from build123d import *

# Parameters (mm, degrees)
SKETCH1_W           = 50.8
SKETCH1_H           = 95.25
BOSS_EXTRUDE1_DEPTH = 38.1
SKETCH2_W           = 74.255386752
SKETCH2_H           = 8.89
F_0_DEG_SLOT_DEPTH  = 19.05
SKETCH3_W           = 5.0292
SKETCH3_H           = 76.2
BOSS_EXTRUDE2_DEPTH = 6.35
SKETCH4_R           = 4.9022
CUT_EXTRUDE2_DEPTH  = 67.067470248
SKETCH5_R           = 5.842
CUT_EXTRUDE3_DEPTH  = 12.319
F_45DEG_SLOT_DEPTH  = 19.05
F_30_DEG_SLOT_DEPTH = 19.05
FILLET2_R           = 6.35
F_15_DEG_SLOT_DEPTH = 19.05
FILLET4_R           = 2.5146
FILLET3_R           = 1.27


with BuildPart() as part:
    # Sketch1 → Boss-Extrude1 (new body)
    with BuildSketch(Plane.XY):
        Rectangle(SKETCH1_W, SKETCH1_H)
    extrude(amount=BOSS_EXTRUDE1_DEPTH)

    # Sketch2 → 0 deg slot (cut)
    with BuildSketch(Plane.XY.offset(38.1)):
        Rectangle(SKETCH2_W, SKETCH2_H)
    extrude(amount=-F_0_DEG_SLOT_DEPTH, mode=Mode.SUBTRACT)

    # Sketch3 → Boss-Extrude2 (add)
    with BuildSketch(Plane(origin=(0, 0, 0), x_dir=(-1, 0, 0), z_dir=(0, 0, -1))):
        with Locations((-15, 0)):
            Rectangle(SKETCH3_W, SKETCH3_H)
    extrude(amount=BOSS_EXTRUDE2_DEPTH)

    # Sketch4 → Cut-Extrude2 (cut, through all)
    with BuildSketch(Plane(origin=(0, 0, 0), x_dir=(-1, 0, 0), z_dir=(0, 0, -1))):
        with Locations((15, 28.575)):
            Circle(SKETCH4_R)
        with Locations((15, -38.1)):
            Circle(SKETCH4_R)
    extrude(amount=-CUT_EXTRUDE2_DEPTH, mode=Mode.SUBTRACT)

    # Sketch5 → Cut-Extrude3 (cut)
    with BuildSketch(Plane.XY.offset(38.1)):
        with Locations((-15, -38.1)):
            Circle(SKETCH5_R)
        with Locations((-15, 28.575)):
            Circle(SKETCH5_R)
    extrude(amount=-CUT_EXTRUDE3_DEPTH, mode=Mode.SUBTRACT)

    # Sketch6 → 45deg slot (cut)
    with BuildSketch(Plane.XY.offset(38.1)):
        Polygon((42.977263594, 49.263442879), (-49.263442879, -42.977263594), (-42.977263594, -49.263442879), (49.263442879, 42.977263594), align=None)
    extrude(amount=-F_45DEG_SLOT_DEPTH, mode=Mode.SUBTRACT)

    # Sketch7 → 30 deg slot (cut)
    with BuildSketch(Plane.XY.offset(38.1)):
        Polygon((48.969673612, 7.869701865), (-53.414673612, 66.981332296), (-48.969673612, 74.680298135), (53.414673612, 15.568667704), align=None)
    extrude(amount=-F_30_DEG_SLOT_DEPTH, mode=Mode.SUBTRACT)

    # Fillet2
    fillet2_edges = [part.edges().sort_by_distance(p)[0] for p in [
        (-25.4, -47.625, 19.05),
        (25.4, -47.625, 19.05),
        (25.4, 47.625, 19.05),
        (-25.4, 47.625, 19.05),
    ]]
    fillet(fillet2_edges, radius=FILLET2_R)

    # Sketch10 → 15 deg slot (cut)
    with BuildSketch(Plane.XY.offset(38.1)):
        Polygon((55.707123796, -8.725123788), (-53.406222485, -37.961956807), (-55.707123796, -29.374876212), (53.406222485, -0.138043193), align=None)
    extrude(amount=-F_15_DEG_SLOT_DEPTH, mode=Mode.SUBTRACT)

    # Fillet4
    fillet4_edges = [part.edges().sort_by_distance(p)[0] for p in [
        (12.4854, 38.1, -3.175),
        (17.5146, 38.1, -3.175),
        (17.5146, -38.1, -3.175),
        (12.4854, -38.1, -3.175),
    ]]
    fillet(fillet4_edges, radius=FILLET4_R - 0.0001)  # a hair under: the kernel refuses the full size

    # Fillet3
    fillet3_edges = [part.edges().sort_by_distance(p)[0] for p in [
        (18.928057645, 25.21423693, 28.575),
        (-2.108522628, 47.625, 28.575),
        (25.4, 31.742947056, 28.575),
        (-19.809556788, 47.579409051, 28.575),
        (-23.721882631, -30.008061916, 28.575),
        (-11.149524062, -17.435703346, 28.575),
        (25.4, -7.64228789, 28.575),
        (25.4, -16.845893134, 28.575),
        (25.4, -4.445, 28.575),
        (-25.4, -4.445, 28.575),
        (25.4, 4.445, 28.575),
        (-25.4, 4.445, 28.575),
        (10.731179285, 4.445, 28.575),
        (-1.841179285, 4.445, 28.575),
        (-25.4, -19.113820715, 28.575),
        (-10.731179285, -4.445, 28.575),
        (25.4, 19.113820715, 28.575),
        (-25.4, -31.686179285, 28.575),
        (1.841179285, -4.445, 28.575),
    ]]
    fillet(fillet3_edges, radius=FILLET3_R)


solid = part.part
For this review, take the finished solid that the model builds, in its own axes (mm). A direction names the side the tool comes from. Round coordinates to 2 decimals unless told otherwise and drop trailing zeros. Loops run counter-clockwise (first coordinate to the right, second up) from the corner with the lowest first, then second, coordinate; pieces in that order, holes last. Notation, with made-up numbers: (12.5, 21.25) - (49.5, 21.25) arc R29 ccw to (49.5, 55.25) - close; hole circle Ø5 at (66.25, -10.5). An arc over 180 degrees is marked (long way). Use one line per item in the form item = value.
1) We need section B-B on x = -15. State how many separate pieces and enclosed holes the cut face has, then the cut area to 3 significant figures.
Solutions:
separate_pieces = 3
enclosed_holes = 0
area = 2,250 mm2
2) We need section D-D on z = 8.5. Write out the cut boundary in (x, y) (3 decimals), then the cut area to 3 significant figures.
Solutions:
outline = (-25.4, -41.275) arc R6.35 ccw to (-19.05, -47.625) - (19.05, -47.625) arc R6.35 ccw to (25.4, -41.275) - (25.4, 41.275) arc R6.35 ccw to (19.05, 47.625) - (-19.05, 47.625) arc R6.35 ccw to (-25.4, 41.275) - close; hole circle Ø9.804 at (-15, -38.1); hole circle Ø9.804 at (-15, 28.575)
area = 4,650 mm2
3) Mouldability with a two-part tool opening along X and no side actions: class faces 6 (the face through (-20, -9, 38.1)), 7 (the face through (18.117, 25.124, 28.442)), 8 (the face through (-17.993, -11.707, 28.708)), 9 (the face through (-23.589, 45.715, 19.317)) as pulls with the +X half, pulls with the -X half, needs draft (parallel to the pull), parting line crosses it, or undercut.
Solutions:
face_6 = needs draft
face_7 = pulls with the +X half
face_8 = undercut
face_9 = pulls with the -X half
4) Tool access review of faces 1 (the face through (-13.937, -42.886, 12.71)), 2 (the face through (-19, -4.445, 29)), 3 (the face through (12.595, 39.136, 28.708)), 4 (the face through (12.485, 0, -3)), 5 (the face through (17.515, 0, -3)): name each direction out of +Z, -Z, +X, -X, +Y, -Y from which nothing blocks a thin tool from reaching the whole face with its end or side.
Solutions:
face_1 = +Z, -Z
face_2 = +Z, +X, -X
face_3 = +Z
face_4 = -Z, -X, +Y, -Y
face_5 = -Z, +X, +Y, -Y
5) Wall thickness on probe 1 along Y at (x, z) = (-15, 11) (3 decimals); probe 2 along X at (y, z) = (-38, 32); probe 3 along Y at (x, z) = (16, 36.5) (3 decimals): over which ranges is each line inside the solid? List them lowest first.
Solutions:
probe_1 = -47.625 to -43.002, -33.198 to 23.673, 33.477 to 47.625
probe_2 = -25.4 to -20.84, -9.16 to 25.4
probe_3 = -47.625 to -19.365, -10.161 to -4.445, 4.445 to 9.714, 22.286 to 26.905, 37.17 to 47.625
6) Clearance check with flat-ended pins moving along their axes: P1, Ø5, axis at x = -10, y = 11.5, coming from the -Z side; P2, Ø3, axis at x = 21.5, z = 26, coming from the -Y side; P3, Ø2, axis at x = -12, y = -21, coming from the +Z side. State where each tip first meets the part, or that it passes through.
Solutions:
P1 = 0
P2 = -47.55
P3 = 19.05
7) We need section C-C on y = 40. Write out the cut boundary in (x, z), then the cut area to 3 significant figures.
Solutions:
outline = (-25.4, 0) - (25.4, 0) - (25.4, 38.1) - (11.1, 38.1) - (11.1, 19.05) - (-6.68, 19.05) - (-6.68, 38.1) - (-25.4, 38.1) - close
area = 1,600 mm2
